For this review, take the finished solid that the model builds, in its own axes (mm). Face numbers are marked on the shaded views. Coordinates: 2 decimals unless noted, no trailing zeros. Order: outer loops, then holes, each group sorted by start corner. A loop starts at its lowest first (then second) coordinate and runs counter-clockwise, first axis right, second up. Notation, with made-up numbers: (73, 35.5) -> (126, 35.5) arc R14 ccw to (126, 39.5) -> close; hole circle Ø9 at (-28, -32.75). An arc over 180 degrees is marked (long way). Return JSON: item names as keys, results as strings. Group by question number.
Item 1: Take a section at B-B (x = -1). Write out the cut boundary in (y, z), then the cut area to 3 significant figures.
Item 2: Take a section at A-A (z = 0). Write out the cut boundary in (x, y), then the cut area to 3 significant figures.
Item 3: Insertion check: pin 1 (1.5 mm diameter, centred on x = 7.5, y = 2.5, fed in from -Z); pin 2 (1 mm diameter, centred on y = 0, z = -10, fed in from +X); pin 3 (1.5 mm diameter, centred on x = 9, z = -3.5, fed in from -Y); pin 4 (1.5 mm diameter, centred on y = 3, z = 11.5, fed in from +X). Each pin has a flat end and moves straight along its axis. Give the tip position at first contact, or say it passes through.
Item 4: Draft analysis for pull direction Z (two halves, no side actions). For the marked faces 1 and 2, state which applies: +Z half, -Z half, draft (parallel to the pull), parting line (faces both ways), or undercut.
Item 5: For line 1 along X through (y, z) = (-0.15, -1); line 2 along Y through (x, z) = (-8.5, -10.5); line 3 along Z through (x, y) = (-6.5, 2), list the stretches that pass through material, from the lowest coordinate up.
Item 6: Take a section at C-C (y = 3.15). Write out the cut boundary in (x, z), then the cut area to 3 significant figures.
Item 7: Take a section at D-D (z = -7). Write out the cut boundary in (x, y).
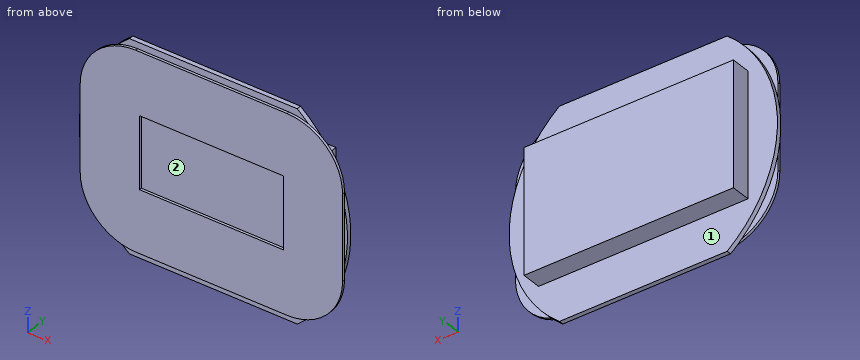
```python
from build123d import *

# Parameters (mm, degrees)
EXTRUDE_1_DEPTH = 0.7
SKETCH_2_W      = 22
SKETCH_2_H      = 11
EXTRUDE_2_DEPTH = 0.4
SKETCH_3_W      = 32
SKETCH_3_H      = 19
EXTRUDE_3_DEPTH = 3


with BuildPart() as part:
    # Эскиз1 → Бобышка-Вытянуть1 (new body)
    with BuildSketch(Plane(origin=(0, 0, 0), x_dir=(1, 0, 0), z_dir=(0, 1, 0))):
        with BuildLine():
            Line((-12.816005618, 16), (12.816005618, 16))
            ThreePointArc((12.816005618, 16), (20.5, 0), (12.816005618, -16))
            Line((12.816005618, -16), (-12.816005618, -16))
            ThreePointArc((-12.816005618, -16), (-20.5, 0), (-12.816005618, 16))
        make_face()
    extrude(amount=EXTRUDE_1_DEPTH)

    # Эскиз2 → Бобышка-Вытянуть2 (add)
    with BuildSketch(Plane.XZ):
        with BuildLine():
            Line((-11.55, 15), (11.55, 15))
            ThreePointArc((11.55, 15), (17.56040764, 12.51040764), (20.05, 6.5))
            Line((20.05, 6.5), (20.05, -6.5))
            ThreePointArc((20.05, -6.5), (17.56040764, -12.51040764), (11.55, -15))
            Line((11.55, -15), (-11.55, -15))
            ThreePointArc((-11.55, -15), (-17.56040764, -12.51040764), (-20.05, -6.5))
            Line((-20.05, -6.5), (-20.05, 6.5))
            ThreePointArc((-20.05, 6.5), (-17.56040764, 12.51040764), (-11.55, 15))
        make_face()
        Rectangle(SKETCH_2_W, SKETCH_2_H, mode=Mode.SUBTRACT)
    extrude(amount=EXTRUDE_2_DEPTH)

    # Эскиз3 → Бобышка-Вытянуть3 (add)
    with BuildSketch(Plane(origin=(0, 0.7, 0), x_dir=(1, 0, 0), z_dir=(0, 1, 0))):
        Rectangle(SKETCH_3_W, SKETCH_3_H)
    extrude(amount=EXTRUDE_3_DEPTH)


solid = part.part
```
Findings below:
{
 "1": {"outline": "(-0.4, -15) -> (0, -15) -> (0, -16) -> (0.7, -16) -> (0.7, -9.5) -> (3.7, -9.5) -> (3.7, 9.5) -> (0.7, 9.5) -> (0.7, 16) -> (0, 16) -> (0, 15) -> (-0.4, 15) -> (-0.4, 5.5) -> (0, 5.5) -> (0, -5.5) -> (-0.4, -5.5) -> close", "area": "87.0 mm2"},
 "2": {"outline": "(-20.5, 0) -> (-20.05, 0) -> (-20.05, -0.4) -> (-11, -0.4) -> (-11, 0) -> (11, 0) -> (11, -0.4) -> (20.05, -0.4) -> (20.05, 0) -> (20.5, 0) -> (20.5, 0.7) -> (16, 0.7) -> (16, 3.7) -> (-16, 3.7) -> (-16, 0.7) -> (-20.5, 0.7) -> close", "area": "132 mm2"},
 "3": {"pin 1": "stops at z = -9.5", "pin 2": "stops at x = 19.5", "pin 3": "stops at y = 0", "pin 4": "passes through"},
 "4": {"face 1": "draft", "face 2": "undercut"},
 "5": {"line 1": "x = -20.05 to -11, 11 to 20.05", "line 2": "y = -0.4 to 0.7", "line 3": "z = -9.5 to 9.5"},
 "6": {"outline": "(-16, -9.5) -> (16, -9.5) -> (16, 9.5) -> (-16, 9.5) -> close", "area": "608 mm2"},
 "7": {"outline": "(-20.04, -0.4) -> (20.04, -0.4) -> (20.04, 0) -> (19.27, 0) -> (19.27, 0.7) -> (16, 0.7) -> (16, 3.7) -> (-16, 3.7) -> (-16, 0.7) -> (-19.27, 0.7) -> (-19.27, 0) -> (-20.04, 0) -> close"}
}
